For this review, take the finished solid that the model builds, in its own axes (mm). A direction names the side the tool comes from. Give positions to 0.01 mm unless a question says otherwise; leave off trailing zeros. Loops run counter-clockwise (first coordinate to the right, second up) from the corner with the lowest first, then second, coordinate; pieces in that order, holes last. Notation, with made-up numbers: M -5,24.25 L 52,24.25 A26 ccw 52,59.25 Z; hole C -23,59 d6. An arc over 180 degrees is marked long. Use CSV: the item, a comma, the result in double quotes. Start each with the question number.
1. To check wall thickness, follow line 1 (X direction, y = -43, z = 44.5); line 2 (X direction, y = -47, z = 61.5); line 3 (Z direction, x = -44.75, y = -48.25). State the ranges of each line that lie inside material, in increasing order. Write a range as [from, to].
2. The part is to be moulded in two halves that separate along Y. For faces 1 (the face through (-32, -44, 63.5)), 2 (the face through (-26.3, -51.54, 44.18)), 3 (the face through (-41.763, -39.949, 44.183)), say which applies: pulls with the +Y half, pulls with the -Y half, needs draft (parallel to the pull), parting line crosses it, or undercut.
3. Tool access review of faces 4 (the face through (-39.503, -32.959, 18.93)), 5 (the face through (-38.242, -51.363, 44.183)), 6 (the face through (-25.54, -52.56, 18.33)): name each direction out of +Z, -Z, +X, -X, +Y, -Y from which nothing blocks a thin tool from reaching the whole face with its end or side.
4. Take a section at B-B, the plane y = -43. Write out the cut boundary in (x, z), and give its area (3 significant figures).
5. Take a section at D-D, the plane z = 49. Write out the cut boundary in (x, y), and give its area (3 significant figures).
6. Take a section at C-C, the plane x = -36.5. Write out the cut boundary in (y, z).
7. Take a section at A-A, the plane z = 10. Write out the cut boundary in (x, y), and give its area (3 significant figures).
8. Insertion check: P1, Ø6, axis at y = -55.5, z = 20.5, coming from the +X side; P2, Ø1, axis at x = -35.5, y = -51.5, coming from the -Z side; P3, Ø4, axis at y = -41, z = 15.5, coming from the -X side; P4, Ø5, axis at y = -53, z = 34.5, coming from the -X side. Each pin has a flat end and moves straight along its axis. Give the tip position at first contact, or say it passes through.
from build123d import *

# Parameters (mm, degrees)
F1_DEPTH = 12.7
F2_SIZE  = 1.27
F3_DEPTH = 12.7
F4_SIZE  = 1.27
F5_DEPTH = 38.1
F6_SIZE  = 2.54


# Not quite as in the source:
# - two fillets or chamfers of one size are made in one step
# - a feature of the source that left no trace in its solid (it failed there, or was rolled back) is left out


with BuildPart() as f1:
    # F0 (on Top) → F1 (new body)
    with BuildSketch(Plane.XY):
        Polygon((-32.2221838869, -58.9305205708), (-17.2413629738, -48.1540753293), (-22.8610431915, -30.5763632619), (-41.315017485, -30.4891850014), (-47.1005206082, -48.0130179407), align=None)
    extrude(amount=F1_DEPTH)

    # F2
    f2_edges = [f1.edges().sort_by_distance(p)[0] for p in [
        (-39.661352, -53.471769, 12.7),
        (-24.731773, -53.542298, 12.7),
        (-20.051203, -39.365219, 12.7),
        (-32.08803, -30.532774, 12.7),
        (-44.207769, -39.251101, 12.7),
    ]]
    chamfer(f2_edges, length=F2_SIZE)

    # F3 (add): a face of the model
    f3_faces = [f1.faces().sort_by_distance(p)[0] for p in [
        (-32.1480256291, -43.2326324208, 12.7),
    ]]
    extrude(f3_faces, amount=F3_DEPTH)

    # F4
    f4_edges = [f1.edges().sort_by_distance(p)[0] for p in [
        (-38.91002, -52.447856, 25.4),
        (-43.001795, -39.649255, 25.4),
        (-25.473399, -52.511331, 25.4),
        (-32.09403, -31.80276, 25.4),
        (-21.260885, -39.751961, 25.4),
    ]]
    chamfer(f4_edges, length=F4_SIZE)

    # F5 (add): a face of the model
    f5_faces = [f1.faces().sort_by_distance(p)[0] for p in [
        (-32.1480256291, -43.2326324208, 25.4),
    ]]
    extrude(f5_faces, amount=F5_DEPTH)

    # F6
    f6_edges = [f1.edges().sort_by_distance(p)[0] for p in [
        (-45.605271, -47.534979, 18.415),
        (-32.214768, -57.360732, 18.415),
        (-40.398318, -31.76353, 18.415),
        (-18.732029, -47.661931, 18.415),
        (-23.789741, -31.84199, 18.415),
    ]]
    chamfer(f6_edges, length=F6_SIZE)


solid = f1.part
Result set:
1,line 1,"[-42.77, -21.56]"
1,line 2,"[-44.09, -20.28]"
1,line 3,"[0, 12.63]"
2,face 1,"needs draft"
2,face 2,"pulls with the -Y half"
2,face 3,"pulls with the +Y half"
3,face 4,"+Z, -X, +Y"
3,face 5,"+Z, -X, -Y"
3,face 6,"+Z, +X, -Y"
4,outline,"M -45.45,0 L -18.89,0 L -18.89,11.43 L -20.22,12.7 L -20.22,24.13 L -21.56,25.4 L -21.56,63.5 L -42.77,63.5 L -42.77,25.4 L -44.11,24.13 L -44.11,12.7 L -45.45,11.43 Z"
4,area,"1,450 mm2"
5,outline,"M -44.11,-47.06 L -32.21,-55.79 L -20.22,-47.17 L -24.72,-33.11 L -39.48,-33.04 Z"
5,area,"375 mm2"
6,outline,"M -55.79,0 L -30.51,0 L -30.51,11.43 L -31.78,12.7 L -31.78,24.13 L -33.05,25.4 L -33.05,63.5 L -52.64,63.5 L -52.64,25.4 L -54.22,24.13 L -54.22,12.7 L -55.79,11.43 Z"
7,outline,"M -47.1,-48.01 L -32.22,-58.93 L -17.24,-48.15 L -22.86,-30.58 L -41.32,-30.49 Z"
7,area,"586 mm2"
8,P1,"x = -25.46"
8,P2,"z = 0"
8,P3,"x = -44.11"
8,P4,"x = -39.42"
